Work out the finished part from the listing and answer in its coordinate system (mm). A direction names the side the tool comes from. Round coordinates to 2 decimals unless told otherwise and drop trailing zeros. Order: outer loops, then holes, each group sorted by start corner. A loop starts at its lowest first (then second) coordinate and runs counter-clockwise, first axis right, second up. Notation, with made-up numbers: (62, 85.5) - (103, 85.5) arc R26 cw to (103, 110.5) - close; hole circle Ø11 at (64.5, -29.75). An arc over 180 degrees is marked (long way). Put each result on its own line as item: value.
Autodesk Inventor part; units mm, degrees
ref_plane "YZ Plane" through (0, 0, 0) normal (1, 0, 0) x (0, 1, 0)
ref_plane "XZ Plane" through (0, 0, 0) normal (0, 1, 0) x (-1, 0, 0)
ref_plane "XY Plane" through (0, 0, 0) normal (0, 0, 1) x (1, 0, 0)
sketch "Эскиз1" plane through (0, 0, 0) normal (1, 0, 0) x (0, 1, 0)
  line L0 (-7.5, -32.85) -> (7.5, -32.85)
  line L1 (7.5, -32.85) -> (7.5, 32.85)
  line L2 (7.5, 32.85) -> (-7.5, 32.85)
  line L3 (-7.5, 32.85) -> (-7.5, -32.85)
  line L4 (-7.5, -32.85) -> (7.5, 32.85) construction
  line L5 (7.5, -32.85) -> (-7.5, 32.85) construction
  line L6 (0, -32.85) -> (0, -16.55) construction
  line L7 (3.3, 4.25) -> (-3.3, 4.25)
  line L8 (-3.3, 4.25) -> (-3.3, -16.55)
  line L9 (-3.3, -16.55) -> (3.3, -16.55)
  line L10 (3.3, -16.55) -> (3.3, 4.25)
  line L11 (7.5, 32.85) -> (-7.5, 32.85)
  line L12 (-7.5, 32.85) -> (-7.5, 10.35)
  line L13 (-7.5, 10.35) -> (7.5, 10.35)
  line L14 (7.5, 10.35) -> (7.5, 32.85)
  line L15 (0, -32.85) -> (-7.5, -12.2439)
  line L16 (0, -32.85) -> (21.9285, -32.85) construction
  point P0 (0, 0)
  point P1 (7.5, 10.35)
  dimension "d0" = 15
  dimension "d1" = 65.7
  dimension "d2" = 16.3
  dimension "d3" = 6.6
  dimension "d4" = 20.8
  dimension "d5" = 22.5
  dimension "d25" = 110
extrude "Выдавливание1" add sketch "Эскиз1" along normal blind 2 contours L3 L15 L0 | L15 L3 L13 L1 L0 | L3 L2 L1 L13 | L10 L9 L8 L7
extrude "Выдавливание2" add sketch "Эскиз1" against normal blind 11.3 contours L10 L9 L8 L7
extrude "Выдавливание3" cut sketch "Эскиз1" along normal blind 0.5 contours L3 L2 L1 L13
chamfer "Фаска2" distance 10.5 angle 45 1 edges at (1.25, -7.5, 32.85)
sketch "Эскиз2" plane through (2, 0, 0) normal (1, 0, 0) x (0, 0, -1)
  line L0 (-22.35, -7.5) -> (-32.85, 3)
  line L1 (-22.35, -7.5) -> (32.85, -7.5)
  line L2 (32.85, -7.5) -> (32.85, 7.5)
  line L3 (32.85, 7.5) -> (-32.85, 7.5)
  line L4 (-32.85, 7.5) -> (-32.85, 3)
  line L5 (31.85, -6.5) -> (-21.9358, -6.5)
  line L6 (-21.9358, -6.5) -> (-31.85, 3.4142)
  line L7 (-31.85, 3.4142) -> (-31.85, 6.5)
  line L8 (-31.85, 6.5) -> (31.85, 6.5)
  line L9 (31.85, 6.5) -> (31.85, -6.5)
  line L10 (-21.5216, -5.5) -> (30.85, -5.5)
  line L11 (30.85, -5.5) -> (30.85, 5.5)
  line L12 (30.85, 5.5) -> (-30.85, 5.5)
  line L13 (-30.85, 5.5) -> (-30.85, 3.8284)
  line L14 (-30.85, 3.8284) -> (-21.5216, -5.5)
  point P0 (0, 0)
  dimension "d27" = 1
  dimension "d33" = 1
extrude "Выдавливание5" cut sketch "Эскиз2" against normal blind 0.4 contours L5 L6 L7 L8 L9
sketch "Эскиз3" plane through (-11.3, 3.3, -16.55) normal (0, 1, 0) x (1, 0, 0)
  line L0 (0, 0) -> (0, -20.8)
  line L1 (0, 0) -> (6.1, 0) construction
  line L2 (6.1, 0) -> (6.1, -10.4) construction
  line L3 (6.1, -10.4) -> (0, -10.4) construction
  line L4 (0, -10.4) -> (0, 0) construction
  circle A0 centre (6.1, -10.4) radius 1.75
  point P0 (11.3, -16.55)
  dimension "d28" = 6.1
  dimension "d29" = 10.4
  dimension "d30" = 3.5
extrude "Выдавливание6" cut sketch "Эскиз3" against normal blind 5
properties part number "switch_cap"
1) Straight lines are drawn through the part: L1, parallel to Z at x = -5.2, y = 2.25; L2, parallel to X at y = -0.35, z = -6.15; L3, parallel to X at y = -6.25, z = 10. For each, find the intervals that lie inside material, in ascending order. Write a range as from..to.
Findings below:
L1: z = -16.55..-7.9, -4.4..4.25
L2: x = -11.3..-6.95, -3.45..2
L3: x = 0..1.6
2) Given pin 1 Ø7.5 at (x, y) = (-4, 0) entering from -Z; pin 2 Ø4 at (y, z) = (-4, -21.5) entering from -X; pin 3 Ø3.5 at (x, z) = (-5.5, -8) entering from +Y; pin 4 Ø2 at (x, z) = (-2.5, -20.5) entering from +Y, each flat-ended and moving along its own axis, determine where each tip first touches the part or whether it passes through.
Findings below:
pin 1: stops at z = -16.55
pin 2: stops at x = 0
pin 3: stops at y = 3.3
pin 4: passes through
3) For faces 4 (the flat face through (-6, -3.3, -6)), 5 (the flat face through (-6, 0, 4.25)), 6 (the flat face through (1.8, -0.77, 26.25)), determine the directions among +Z, -Z, +X, -X, +Y, -Y from which every point of the face is accessible in a straight line to the end or side of a thin tool.
Findings below:
face 4: +Z, -Z, -X, -Y
face 5: +Z, -X, +Y, -Y
face 6: +X
4) A cutting plane is placed at C-C on y = 0. Write down the section's boundary in (x, z).
Findings below:
outline: (-11.3, -16.55) - (0, -16.55) - (0, -32.85) - (2, -32.85) - (2, -31.85) - (1.6, -31.85) - (1.6, -30.85) - (2, -30.85) - (2, 27.02) - (1.6, 27.02) - (1.6, 28.44) - (2, 28.44) - (2, 29.85) - (0.5, 29.85) - (0.5, 10.35) - (0, 10.35) - (0, 4.25) - (-11.3, 4.25) - close; hole circle Ø3.5 at (-5.2, -6.15)
5) A cutting plane is placed at A-A on z = 11. Write down the section's boundary in (x, y).
Findings below:
outline: (0.5, -7.5) - (2, -7.5) - (2, -6.5) - (1.6, -6.5) - (1.6, -5.5) - (2, -5.5) - (2, 5.5) - (1.6, 5.5) - (1.6, 6.5) - (2, 6.5) - (2, 7.5) - (0.5, 7.5) - close
6) A cutting plane is placed at B-B on x = -6. Write down the section's boundary in (y, z), then the cut area to 3 significant figures.
Findings below:
outline: (-3.3, -16.55) - (3.3, -16.55) - (3.3, -7.71) - (-1.7, -7.71) - (-1.7, -4.59) - (3.3, -4.59) - (3.3, 4.25) - (-3.3, 4.25) - close
area: 122 mm2
7) A cutting plane is placed at D-D on z = -6.15. Write down the section's boundary in (x, y).
Findings below:
outline: (-11.3, -3.3) - (0, -3.3) - (0, -7.5) - (2, -7.5) - (2, -6.5) - (1.6, -6.5) - (1.6, -5.5) - (2, -5.5) - (2, 5.5) - (1.6, 5.5) - (1.6, 6.5) - (2, 6.5) - (2, 7.5) - (0, 7.5) - (0, 3.3) - (-3.45, 3.3) - (-3.45, -1.7) - (-6.95, -1.7) - (-6.95, 3.3) - (-11.3, 3.3) - close
8) For a pull along Y with two mould halves and no side action, classify faces 1 (the flat face through (1.803, -1.612, 26.824)), 2 (the flat face through (0.5, 0, 19)), 3 (the flat face through (1, 7.5, 0)) as pulls with the +Y half, pulls with the -Y half, needs draft (parallel to the pull), parting line crosses it, or undercut.
Findings below:
face 1: undercut
face 2: needs draft
face 3: pulls with the +Y half
